Here's how the part is built. I have some questions about the finished solid (model axes, mm). Face numbers are marked on the shaded views. A direction names the side the tool comes from. Give positions to 0.01 mm unless a question says otherwise; leave off trailing zeros. Loops run counter-clockwise (first coordinate to the right, second up) from the corner with the lowest first, then second, coordinate; pieces in that order, holes last. Notation, with made-up numbers: (-19.75, 55.5) - (12.25, 55.5) arc R21 ccw to (12.25, 90.5) - close; hole circle Ø1 at (39, 57.25). An arc over 180 degrees is marked (long way). Return JSON: item names as keys, results as strings. Group by question number.
(1) On a 3-axis mill with a long thin cutter (end or side, diameter ignored), from which of +Z, -Z, +X, -X, +Y, -Y can I reach the whole of each face in a straight line? I mean the marked faces 4 and 5. Say none if no direction works.
(2) If we section it at D-D (y = 19.25): Please give me the cut outline in (x, z), then the cut area to 3 significant figures.
(3) If we mould it in two halves opening along X, with no side actions, what happens to the marked faces 1, 2 and 3? For each: released by +X, released by -X, zero draft, split by the parting line, or undercut.
(4) If we section it at B-B (y = 7.5): Please give me the cut outline in (x, z).
(5) For P1, Ø1, axis at x = -8.5, z = -0.5, coming from the +Y side; P2, Ø1.2, axis at y = 9.5, z = -7.5, coming from the +X side, each with a flat end and sliding along its axis, tell me the tip position at first contact or that it passes through.
(6) If we section it at A-A (x = 0): Please give me the cut outline in (y, z).
(7) I need wall thicknesses on probe 1 along X at (y, z) = (13.5, -7.75); probe 2 along Y at (x, z) = (21.45, 7.5); probe 3 along Y at (x, z) = (21.4, 0). Which ranges of each line are inside material? Lowest first, please. Write a range as [from, to].
(8) If we section it at C-C (z = 7.5): Please give me the cut outline in (x, y).
```python
from build123d import *

# Parameters (mm, degrees)
SKETCH_1_W          = 40
SKETCH_1_H          = 20
SKETCH_1_R          = 3
SKETCH_1_R_2        = 1.5
EXTRUDE_1_DEPTH     = 2
SKETCH_2_W          = 2
SKETCH_2_H          = 20
EXTRUDE_2_DEPTH     = 27
SKETCH_3_R          = 4
SKETCH_3_R_2        = 1
CUT_EXTRUDE_1_DEPTH = 22
SKETCH_4_R          = 4
SKETCH_4_R_2        = 1
CUT_EXTRUDE_2_DEPTH = 37.235341864
FILLET_1_R          = 2
FILLET_2_R          = 1


with BuildPart() as part:
    # 草图1 → 凸台-拉伸1 (new body)
    with BuildSketch(Plane(origin=(0, 0, 0), x_dir=(1, 0, 0), z_dir=(0, 1, 0))):
        Rectangle(SKETCH_1_W, SKETCH_1_H)
        with Locations(Location((0, 0, 0), (0, 0, 270))):
            Circle(SKETCH_1_R, mode=Mode.SUBTRACT)
        with Locations(Location((-4.949747468, -4.949747468, 0), (0, 0, 270))):
            Circle(SKETCH_1_R_2, mode=Mode.SUBTRACT)
        with Locations(Location((-4.949747468, 4.949747468, 0), (0, 0, 270))):
            Circle(SKETCH_1_R_2, mode=Mode.SUBTRACT)
        with Locations(Location((4.949747468, 4.949747468, 0), (0, 0, 270))):
            Circle(SKETCH_1_R_2, mode=Mode.SUBTRACT)
        with Locations(Location((4.949747468, -4.949747468, 0), (0, 0, 270))):
            Circle(SKETCH_1_R_2, mode=Mode.SUBTRACT)
    extrude(amount=EXTRUDE_1_DEPTH)

    # 草图2 → 凸台-拉伸2 (add)
    with BuildSketch(Plane(origin=(0, 0, 0), x_dir=(1, 0, 0), z_dir=(0, 1, 0))):
        with Locations((21, 0)):
            Rectangle(SKETCH_2_W, SKETCH_2_H)
        with Locations((-21, 0)):
            Rectangle(SKETCH_2_W, SKETCH_2_H)
    extrude(amount=EXTRUDE_2_DEPTH)

    # 草图3 → 切除-拉伸1 (cut)
    with BuildSketch(Plane(origin=(0, 0, 0), x_dir=(0, 0, -1), z_dir=(1, 0, 0))):
        with BuildLine():
            Line((-10, 27), (-10, 17))
            ThreePointArc((-10, 17), (-7.071067827, 24.071067797), (-4.3e-08, 27))
            Line((-4.3e-08, 27), (-10, 27))
        make_face()
        with BuildLine():
            ThreePointArc((-4.3e-08, 27), (7.071067797, 24.071067827), (10, 17))
            Line((10, 17), (10, 27))
            Line((10, 27), (-4.3e-08, 27))
        make_face()
        with Locations((0, 17)):
            Circle(SKETCH_3_R)
        with Locations((0, 10)):
            Circle(SKETCH_3_R_2)
        with Locations((7, 17)):
            Circle(SKETCH_3_R_2)
        with Locations((0, 24)):
            Circle(SKETCH_3_R_2)
        with Locations((-7, 17)):
            Circle(SKETCH_3_R_2)
    extrude(amount=-CUT_EXTRUDE_1_DEPTH, mode=Mode.SUBTRACT)

    # 草图4 → 切除-拉伸2 (cut, through all)
    with BuildSketch(Plane(origin=(0, 0, 0), x_dir=(0, 0, -1), z_dir=(1, 0, 0))):
        with Locations((0, 17)):
            Circle(SKETCH_4_R)
        with Locations((-7.5, 24.5)):
            Circle(SKETCH_4_R_2)
        with Locations(Location((-7.5, 9.5, 0), (0, 0, 180))):
            Circle(SKETCH_4_R_2)
        with Locations((7.5, 9.5)):
            Circle(SKETCH_4_R_2)
        with Locations(Location((7.5, 24.5, 0), (0, 0, 180))):
            Circle(SKETCH_4_R_2)
    extrude(amount=CUT_EXTRUDE_2_DEPTH, mode=Mode.SUBTRACT)

    # 圆角1
    fillet_1_edges = [part.edges().sort_by_distance(p)[0] for p in [
        (22, 0, 0),
        (-22, 0, 0),
    ]]
    fillet(fillet_1_edges, radius=FILLET_1_R)

    # 圆角2
    fillet_2_edges = [part.edges().sort_by_distance(p)[0] for p in [
        (21, 27, 10),
        (21, 27, -10),
    ]]
    fillet(fillet_2_edges, radius=FILLET_2_R)


solid = part.part
```
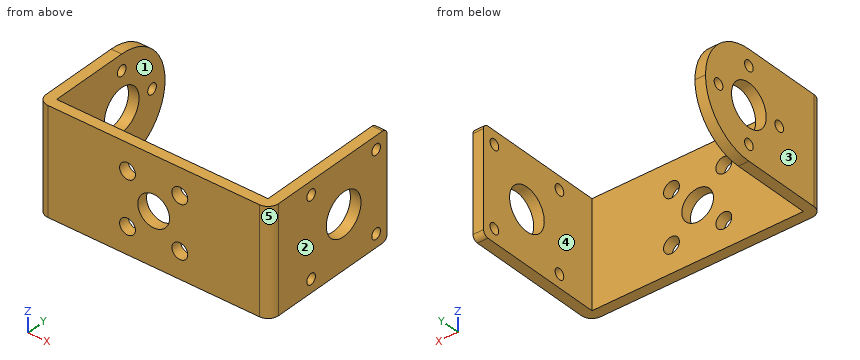
Values:
{
 "1": {"face 4": "+Z, -Z, +Y", "face 5": "+Z, -Z, +X, -Y"},
 "2": {"outline": "(-22, -9.74) - (-20, -9.74) - (-20, -3.31) - (-22, -3.31) - close; (-22, 3.31) - (-20, 3.31) - (-20, 9.74) - (-22, 9.74) - close; (20, -10) - (22, -10) - (22, -3.31) - (20, -3.31) - close; (20, 3.31) - (22, 3.31) - (22, 10) - (20, 10) - close", "area": "52.5 mm2"},
 "3": {"face 1": "undercut", "face 2": "released by +X", "face 3": "released by -X"},
 "4": {"outline": "(-22, -10) - (-20, -10) - (-20, 10) - (-22, 10) - close; (20, -10) - (22, -10) - (22, 10) - (20, 10) - close"},
 "5": {"P1": "y = 2", "P2": "x = -20"},
 "6": {"outline": "(0, -10) - (2, -10) - (2, -3) - (0, -3) - close; (0, 3) - (2, 3) - (2, 10) - (0, 10) - close"},
 "7": {"probe 1": "[-22, -20], [20, 22]", "probe 2": "[0.62, 8.5], [10.5, 23.5], [25.5, 27]", "probe 3": "[0.57, 13], [21, 27]"},
 "8": {"outline": "(-22, 2) arc R2 ccw to (-20, 0) - (20, 0) arc R2 ccw to (22, 2) - (22, 8.5) - (20, 8.5) - (20, 2) - (-20, 2) - (-20, 16.13) - (-22, 16.13) - close; (-22, 17.87) - (-20, 17.87) - (-20, 23.61) - (-22, 23.61) - close; (20, 10.5) - (22, 10.5) - (22, 23.5) - (20, 23.5) - close; (20, 25.5) - (22, 25.5) - (22, 27) - (20, 27) - close"}
}
